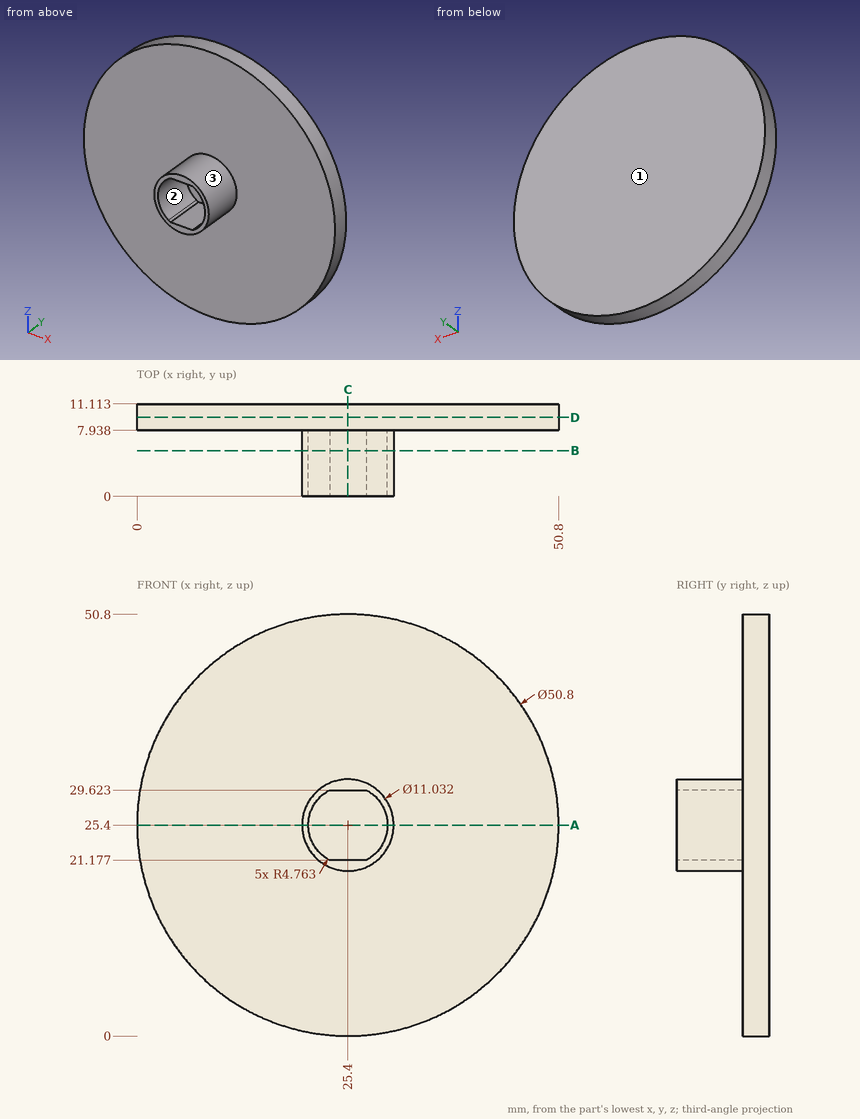
Verification items for this drawing (mm, ordinates from the low corner). Coordinates: 2 decimals unless noted, no trailing zeros. Loops run counter-clockwise (first coordinate to the right, second up) from the corner with the lowest first, then second, coordinate; pieces in that order, holes last. Notation, with made-up numbers: (-25.5, -1.75) - (-9.5, -1.75) arc R28 cw to (-9.5, 26.25) - close; hole circle Ø3 at (-14, 4). An arc over 180 degrees is marked (long way). One line per item, written item: value. Start each with the question number.
(1) Cross-section at A-A on z = 25.4. Enter the section's corners in (x, y).
(2) Material ranges on line 1 (Z direction, x = 25.5, y = 3) (1 decimal); line 2 (X direction, y = 6.25, z = 22.5); line 3 (Y direction, x = 32.5, z = 18.5), recorded low to high. Write a range as [from, to].
(3) Cross-section at B-B on y = 5.5. Enter the section's corners in (x, z) (1 decimal).
(4) Mould release check, pull along X, two halves, no side actions. Record for the marked faces 1, 2 and 3: released by +X, released by -X, zero draft, split by the parting line, or undercut.
(5) Depth check by flat-ended pin: P1, Ø5, axis at x = 25.5, y = 3.5, coming from the -Z side; P2, Ø4, axis at x = 26, z = 26.5, coming from the -Y side; P3, Ø1.5, axis at x = 10.5, y = 9.5, coming from the -Z side (1 decimal). Enter the tip coordinate at first touch or a pass-through.
(6) Cross-section at D-D on y = 9.5. Enter the section's corners in (x, z).
(7) Cross-section at C-C on x = 25.4. Enter the section's corners in (y, z), plus the area to 3 significant figures.
Results below:
1. outline: (0, 7.94) - (19.88, 7.94) - (19.88, 0) - (20.64, 0) - (20.64, 7.94) - (30.16, 7.94) - (30.16, 0) - (30.92, 0) - (30.92, 7.94) - (50.8, 7.94) - (50.8, 11.11) - (0, 11.11) - close
2. line 1: z = [19.9, 21.2], [29.6, 30.9]
2. line 2: x = [20.71, 21.62], [29.18, 30.09]
2. line 3: y = [7.94, 11.11]
3. outline: circle Ø11 at (25.4, 25.4); hole (22.8, 21.4) arc R4.8 ccw to (23.2, 21.2) - (27.6, 21.2) arc R4.8 ccw to (28, 21.4) arc R4.8 ccw to (28, 29.4) arc R4.8 ccw to (27.6, 29.6) - (23.2, 29.6) arc R4.8 ccw to (22.8, 29.4) arc R4.8 ccw to start
4. face 1: zero draft
4. face 2: undercut
4. face 3: split by the parting line
5. P1: stops at z = 19.88
5. P2: stops at y = 7.94
5. P3: stops at z = 4.3
6. outline: circle Ø50.8 at (25.4, 25.4)
7. outline: (0, 19.88) - (7.94, 19.88) - (7.94, 0) - (11.11, 0) - (11.11, 50.8) - (7.94, 50.8) - (7.94, 30.92) - (0, 30.92) - (0, 29.62) - (7.94, 29.62) - (7.94, 21.18) - (0, 21.18) - close
7. area: 182 mm2
